from build123d import *

# Parameters (mm, degrees)
F1_DEPTH = 10.16
F0_R     = 3.3655
F0_W     = 22.5806
F0_H     = 22.4536
F2_DEPTH = 5.08
F3_START = 2.54
F3_DEPTH = 2.54


with BuildPart() as f1:
    # F0 (on Top) → F1 (new body)
    with BuildSketch(Plane.XY):
        Polygon((-44.0307967365, -11.1630027373), (-44.0307967365, -14.2110027373), (152.8192032635, -14.2110027373), (152.8192032635, 17.5389972627), (-44.0307967365, 17.5389972627), (-44.0307967365, 14.4909972627), (149.7712032635, 14.4909972627), (149.7712032635, -11.1630027373), align=None)
    extrude(amount=F1_DEPTH)

    # F0 (on Top) → F2 (join)
    with BuildSketch(Plane.XY):
        Polygon((-44.0307967365, -9.5628027373), (-44.0307967365, -11.1630027373), (149.7712032635, -11.1630027373), (149.7712032635, 14.4909972627), (-44.0307967365, 14.4909972627), (-44.0307967365, 12.8907972627), (-21.4501967365, 12.8907972627), (-21.4501967365, -9.5628027373), align=None)
        with Locations((-12.2807967365, 1.6639972627)):
            Circle(F0_R, mode=Mode.SUBTRACT)
        with Locations((121.0692032635, 1.6639972627)):
            Circle(F0_R, mode=Mode.SUBTRACT)
        with Locations((-32.7404967365, 1.6639972627)):
            Rectangle(F0_W, F0_H)
    extrude(amount=F2_DEPTH)

    # F0 (on Top) → F3 (cut)
    with BuildSketch(Plane.XY.offset(F3_START)):
        with Locations((-32.7404967365, 1.6639972627)):
            Rectangle(F0_W, F0_H)
    extrude(amount=F3_DEPTH, mode=Mode.SUBTRACT)


solid = f1.part
Model file for the job. Use its own axes, mm. A direction names the side the tool comes from. Coordinates: 2 decimals unless noted, no trailing zeros. Loops run counter-clockwise (first coordinate to the right, second up) from the corner with the lowest first, then second, coordinate; pieces in that order, holes last. Notation, with made-up numbers: (86, 3.25) -> (142, 3.25) arc R9 cw to (142, 13.25) -> close; hole circle Ø11 at (-0.5, 79.5). An arc over 180 degrees is marked (long way). Use one line per item in the form item = value. Start each with the question number.
(1) Probe probe 1 along X at (y, z) = (2, 1); probe 2 along Z at (x, y) = (17.5, -6); probe 3 along X at (y, z) = (-4.5, 4.5). List the from-to ranges inside material, lowest first. Write a range as from..to.
(2) Cut at A-A on x = 121.5. Give the cut face in (y, z).
(3) Tool access for faces 4 (the flat face through (152.819, 1, 5)), 5 (the flat face through (149.771, 2, 8)): list every direction of +Z, -Z, +X, -X, +Y, -Y with a clear straight run to the whole face (end or side of a thin tool).
(4) Pull direction Y, two halves, no side cores. Call faces 1 (the flat face through (53, 2, 0)), 2 (the cylindrical face through (117.707, 1.812, 2.504)), 3 (the flat face through (56, 17.539, 5)): pulls with the +Y half, pulls with the -Y half, needs draft (parallel to the pull), parting line crosses it, or undercut.
(5) Cut at C-C on y = 7. Give the cut face in (x, z).
(6) Cut at B-B on z = 7.5. Give the cut face in (x, y).
(7) Cut at D-D on x = -30. Give the cut face in (y, z), and give its area (3 significant figures).
(8) Flat gauge pins, fed straight in: pin 1 (5.5 mm diameter, centred on y = 4, z = 7, fed in from -X); pin 2 (13 mm diameter, centred on x = 78, y = 7, fed in from +Z); pin 3 (1 mm diameter, centred on y = -0.5, z = 7.5, fed in from -X). Where does each tip first touch, or does it go through?
Values:
q1.probe_1 = -44.03..-15.63, -8.93..117.72, 124.42..152.82
q1.probe_2 = 0..5.08
q1.probe_3 = -21.45..152.82
q2.outline = (-14.21, 0) -> (-1.67, 0) -> (-1.67, 5.08) -> (-11.16, 5.08) -> (-11.16, 10.16) -> (-14.21, 10.16) -> close; (5, 0) -> (17.54, 0) -> (17.54, 10.16) -> (14.49, 10.16) -> (14.49, 5.08) -> (5, 5.08) -> close
q3.face_4 = +Z, -Z, +X, +Y, -Y
q3.face_5 = +Z, -X
q4.face_1 = needs draft
q4.face_2 = undercut
q4.face_3 = pulls with the +Y half
q5.outline = (-44.03, 0) -> (152.82, 0) -> (152.82, 10.16) -> (149.77, 10.16) -> (149.77, 5.08) -> (-21.45, 5.08) -> (-21.45, 2.54) -> (-44.03, 2.54) -> close
q6.outline = (-44.03, -14.21) -> (152.82, -14.21) -> (152.82, 17.54) -> (-44.03, 17.54) -> (-44.03, 14.49) -> (149.77, 14.49) -> (149.77, -11.16) -> (-44.03, -11.16) -> close
q7.outline = (-14.21, 0) -> (17.54, 0) -> (17.54, 10.16) -> (14.49, 10.16) -> (14.49, 5.08) -> (12.89, 5.08) -> (12.89, 2.54) -> (-9.56, 2.54) -> (-9.56, 5.08) -> (-11.16, 5.08) -> (-11.16, 10.16) -> (-14.21, 10.16) -> close
q7.area = 135 mm2
q8.pin_1 = -21.45
q8.pin_2 = 5.08
q8.pin_3 = 149.77
